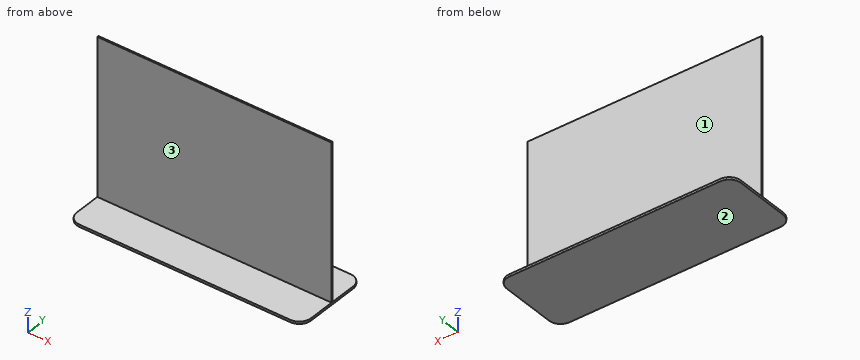
```python
from build123d import *

# Parameters (mm, degrees)
PAD_DEPTH    = 0.6
SKETCH001_W  = 60
SKETCH001_H  = 0.37
PAD001_DEPTH = 40


with BuildPart() as part:
    # Sketch → Pad (new body)
    with BuildSketch(Plane.XY):
        with BuildLine():
            Line((-27, 10), (27, 10))
            ThreePointArc((30, 7), (29.12132, 9.12132), (27, 10))
            Line((30, 7), (30, -7))
            ThreePointArc((27, -10), (29.12132, -9.12132), (30, -7))
            Line((27, -10), (-27, -10))
            ThreePointArc((-30, -7), (-29.12132, -9.12132), (-27, -10))
            Line((-30, -7), (-30, 7))
            ThreePointArc((-27, 10), (-29.12132, 9.12132), (-30, 7))
        make_face()
    extrude(amount=PAD_DEPTH)

    # Sketch001 → Pad001 (join)
    with BuildSketch(Plane.XY.offset(0.6)):
        Rectangle(SKETCH001_W, SKETCH001_H)
    extrude(amount=PAD001_DEPTH)


solid = part.part
```
Here's how the part is built. I have some questions about the finished solid (model axes, mm). Face numbers are marked on the shaded views. A direction names the side the tool comes from. Round coordinates to 2 decimals unless told otherwise and drop trailing zeros. Loops run counter-clockwise (first coordinate to the right, second up) from the corner with the lowest first, then second, coordinate; pieces in that order, holes last.
1. Will these pins go through, and if not, where does the flat tip stop? pin 1 (5 mm diameter, centred on x = 21.5, z = 23.5, fed in from -Y) (3 decimals); pin 2 (8 mm diameter, centred on x = 4, y = 5, fed in from +Z); pin 3 (1 mm diameter, centred on x = -13, z = 25, fed in from +Y) (3 decimals); pin 4 (2 mm diameter, centred on y = 2.5, z = 22, fed in from +X).
Answers:
pin 1: stops at y = -0.185
pin 2: stops at z = 0.6
pin 3: stops at y = 0.185
pin 4: passes through
2. Suppose I cut it at A-A, the plane x = -24.5. Please give me the cut outline in (y, z) (3 decimals).
Answers:
outline: (-10, 0) - (10, 0) - (10, 0.6) - (0.185, 0.6) - (0.185, 40.6) - (-0.185, 40.6) - (-0.185, 0.6) - (-10, 0.6) - close
3. Suppose I cut it at B-B, the plane z = 31. Please give me the cut outline in (x, y) (3 decimals).
Answers:
outline: (-30, -0.185) - (30, -0.185) - (30, 0.185) - (-30, 0.185) - close
4. Suppose I cut it at C-C, the plane y = -5. Please give me the cut outline in (x, z), and give its area (3 significant figures).
Answers:
outline: (-30, 0) - (30, 0) - (30, 0.6) - (-30, 0.6) - close
area: 36.0 mm2
5. For the marked faces 1, 2 and 3, which set-ups out of +Z, -Z, +X, -X, +Y, -Y let a thin tool reach every point of the face, with its end or its side?
Answers:
face 1: +Z, +X, -X, +Y
face 2: -Z, +X, -X, +Y, -Y
face 3: +Z, +X, -X, -Y
6. If I drill on probe 1 along Z at (x, y) = (-17.5, 2); probe 2 along Y at (x, z) = (-3, 2.5) (3 decimals), over which ranges is the centre line in solid material (lowest first)?
Answers:
probe 1: z = 0 to 0.6
probe 2: y = -0.185 to 0.185
